```python
from build123d import *

# Parameters (mm, degrees)
CUT_EXTRUDE1_DEPTH = 4.8


with BuildPart() as part:
    # Sketch1 → Revolve1 (revolve)
    with BuildSketch(Plane.XY, mode=Mode.PRIVATE) as revolve1_sk:
        with BuildLine():
            Line((0, 0), (6, 0))
            ThreePointArc((6, 0), (8.904011689, 1.140264724), (10.151169128, 4))
            Line((10.151169128, 4), (0, 4))
            Line((0, 4), (0, 0))
        make_face()
    revolve(revolve1_sk.sketch.rotate(Axis((0, 4, 0), (0, -1, 0)), 180), axis=Axis((0, 4, 0), (0, -1, 0)))

    # Sketch2 → Cut-Extrude1 (cut)
    with BuildSketch(Plane.XZ):
        Polygon((4, 0), (2, 3.464101615), (-2, 3.464101615), (-4, 0), (-2, -3.464101615), (2, -3.464101615), align=None)
    extrude(amount=-CUT_EXTRUDE1_DEPTH, mode=Mode.SUBTRACT)


solid = part.part
```
Source: CAD feature listing. Evaluate the final solid. Frame: model axes, mm. A direction names the side the tool comes from. Coordinates: 2 decimals unless noted, no trailing zeros. Order: outer loops, then holes, each group sorted by start corner. A loop starts at its lowest first (then second) coordinate and runs counter-clockwise, first axis right, second up. Notation, with made-up numbers: M -33.5,83 L -29.5,83 A17 ccw -29.5,116 Z; hole C 14.5,14.25 d8. An arc over 180 degrees is marked long. Write each question's results on one line, items separated by ' | '. Start each with the question number.
1) Contact query for flat-ended pins moving along their axis: pin 1 Ø2 at (y, z) = (3, -1) entering from +X; pin 2 Ø1.5 at (y, z) = (3.5, -3.5) entering from +X; pin 3 Ø1.5 at (y, z) = (1.5, -3) entering from +X. Output: stop coordinate, or through.
2) Line query: line 1 (X direction, y = 3.6, z = -1.5); line 2 (Z direction, x = -3.5, y = 3.8); line 3 (X direction, y = 0.65, z = -2.5). Output: solid intervals per line, ascending. Write a range as from..to.
3) Section query C-C (y = 3.65). Return the cut outline in (x, z).
4) Access query for faces 3 (the face through (3, 0, 3)), 4 (the face through (-2.986, 1.972, 1.756)). Directions: +Z, -Z, +X, -X, +Y, -Y. A direction counts if a zero-diameter tool reaches every point of the face in a straight line with its end or side. Return the directions, or none.
5) Section query A-A (x = 0). Return the cut outline in (y, z).
6) Section query B-B (y = 0.5). Return the cut outline in (x, z).
7) Draft query along X for faces 1 (the face through (2.986, 1.972, -1.756)), 2 (the face through (-4.4, 4, -0.1)). Return one class per face: released by +X, released by -X, zero draft, split by the parting line, or undercut.
Answers:
1) pin 1: stops at x = 10.13 | pin 2: stops at x = 9.75 | pin 3: stops at x = 9.31
2) line 1: x = -10.01..-3.13, 3.13..10.01 | line 2: z = -9.52..-0.87, 0.87..9.52 | line 3: x = -7.9..-2.56, 2.56..7.9
3) outline: C 0,0 d20.26; hole M -4,0 L -2,-3.46 L 2,-3.46 L 4,0 L 2,3.46 L -2,3.46 Z
4) face 3: +Z, -Z, +X, -X, -Y | face 4: +Y, -Y
5) outline: M 0,-6 A4.08 ccw 4,-10.15 L 4,-3.46 L 0,-3.46 Z; M 0,3.46 L 4,3.46 L 4,10.15 A4.08 ccw 0,6 Z
6) outline: C 0,0 d16.07; hole M -4,0 L -2,-3.46 L 2,-3.46 L 4,0 L 2,3.46 L -2,3.46 Z
7) face 1: undercut | face 2: zero draft
